Source: CAD feature listing. Evaluate the final solid. Frame: model axes, mm. Face numbers are marked on the shaded views. A direction names the side the tool comes from. Coordinates: 2 decimals unless noted, no trailing zeros. Write each loop counter-clockwise with the first axis right and the second up, starting at its lowest first coordinate (ties: lowest second). Pieces come first, ordered by that corner, then holes. Notation, with made-up numbers: M 42,26.25 L 74,26.25 A26 cw 74,50.25 Z; hole C 3,-30 d6. An arc over 180 degrees is marked long. One line per item, written item: value. Start each with the question number.
Item 1: Cut plane A-A, the plane z = 5.5. Output: boundary loops of the cut face in (x, y), then the cut area to 3 significant figures.
Item 2: Set-up query: the marked faces 1, 2, 3 and 4. Return all of +Z, -Z, +X, -X, +Y, -Y with unobstructed straight access to the full face (end or side cutting, diameter ignored); none if empty.
Item 3: Ray query, L1, parallel to X at y = 5.4, z = -7.5; L2, parallel to X at y = 4.3, z = 17.25; L3, parallel to Z at x = 0.5, y = 2.9. Return the intervals inside material, ascending. Write a range as from..to.
Item 4: Pin query (flat end, axial travel): P1, Ø3, axis at y = 5, z = -7, coming from the -X side; P2, Ø0.5, axis at x = -0.5, y = 5, coming from the -Z side; P3, Ø1.3, axis at y = 4.5, z = 1, coming from the +X side. Return the tip coordinate at first contact, or that it passes through.
Item 5: Cut plane C-C, the plane z = -4. Output: boundary loops of the cut face in (x, y).
Item 6: Cut plane B-B, the plane x = 3. Output: boundary loops of the cut face in (y, z), then the cut area to 3 significant figures.
```python
from build123d import *

# Parameters (mm, degrees)
SKETCH1_W           = 15.5
SKETCH1_H           = 11
BOSS_EXTRUDE1_DEPTH = 1.6
BOSS_EXTRUDE2_DEPTH = 1.6
SKETCH3_W           = 40.5
SKETCH3_H           = 21
BOSS_EXTRUDE3_DEPTH = 6
CUT_EXTRUDE1_DEPTH  = 2.6
SKETCH5_W           = 5
SKETCH5_H           = 4
BOSS_EXTRUDE4_DEPTH = 6
LPATTERN1_COUNT     = 2
LPATTERN1_PITCH     = 15
LPATTERN1_COL_COUNT = 2
LPATTERN1_COL_PITCH = 15
SKETCH6_W           = 4
SKETCH6_H           = 5
BOSS_EXTRUDE5_DEPTH = 6
SKETCH7_W           = 2.75
SKETCH7_H           = 4
BOSS_EXTRUDE6_DEPTH = 6


with BuildPart() as part:
    # Sketch1 → Boss-Extrude1 (new body)
    with BuildSketch(Plane(origin=(0, 0, 0), x_dir=(1, 0, 0), z_dir=(0, 1, 0))):
        with Locations((7.75, -5.5)):
            Rectangle(SKETCH1_W, SKETCH1_H)
    extrude(amount=BOSS_EXTRUDE1_DEPTH)

    # Sketch2 → Boss-Extrude2 (add, through all)
    with BuildSketch(Plane(origin=(0, 1.6, 0), x_dir=(1, 0, 0), z_dir=(0, 1, 0))):
        with BuildLine():
            Line((-1.75, -4), (-1.75, -2.6))
            ThreePointArc((-1.75, -2.6), (-4.65, -5.5), (-1.75, -8.4))
            Line((-1.75, -8.4), (-1.75, -7))
            ThreePointArc((-1.75, -7), (-3.25, -5.5), (-1.75, -4))
        make_face()
        with BuildLine():
            ThreePointArc((0, -3.187533784), (-0.827002716, -2.750804479), (-1.75, -2.6))
            Line((-1.75, -2.6), (-1.75, -4))
            ThreePointArc((-1.75, -4), (-0.689339828, -4.439339828), (-0.25, -5.5))
            ThreePointArc((-0.25, -5.5), (-0.689339828, -6.560660172), (-1.75, -7))
            Line((-1.75, -7), (-1.75, -8.4))
            ThreePointArc((-1.75, -8.4), (-0.827002716, -8.249195521), (0, -7.812466216))
            Line((0, -7.812466216), (0, -3.187533784))
        make_face()
        with BuildLine():
            Line((0, -2.6), (-1.75, -2.6))
            ThreePointArc((-1.75, -2.6), (-0.827002716, -2.750804479), (0, -3.187533784))
            Line((0, -3.187533784), (0, -2.6))
        make_face()
        with BuildLine():
            ThreePointArc((0, -7.812466216), (-0.827002716, -8.249195521), (-1.75, -8.4))
            Line((-1.75, -8.4), (0, -8.4))
            Line((0, -8.4), (0, -7.812466216))
        make_face()
        with BuildLine():
            ThreePointArc((20.15, -5.5), (19.300609665, -3.449390335), (17.25, -2.6))
            Line((17.25, -2.6), (17.25, -4))
            ThreePointArc((17.25, -4), (18.310660172, -4.439339828), (18.75, -5.5))
            ThreePointArc((18.75, -5.5), (18.310660172, -6.560660172), (17.25, -7))
            Line((17.25, -7), (17.25, -8.4))
            ThreePointArc((17.25, -8.4), (19.300609665, -7.550609665), (20.15, -5.5))
        make_face()
        with BuildLine():
            Line((17.25, -4), (17.25, -2.6))
            ThreePointArc((17.25, -2.6), (16.327002716, -2.750804479), (15.5, -3.187533784))
            Line((15.5, -3.187533784), (15.5, -7.812466216))
            ThreePointArc((15.5, -7.812466216), (16.327002716, -8.249195521), (17.25, -8.4))
            Line((17.25, -8.4), (17.25, -7))
            ThreePointArc((17.25, -7), (15.75, -5.5), (17.25, -4))
        make_face()
        with BuildLine():
            Line((17.25, -2.6), (15.5, -2.6))
            Line((15.5, -2.6), (15.5, -3.187533784))
            ThreePointArc((15.5, -3.187533784), (16.327002716, -2.750804479), (17.25, -2.6))
        make_face()
        with BuildLine():
            Line((15.5, -7.812466216), (15.5, -8.4))
            Line((15.5, -8.4), (17.25, -8.4))
            ThreePointArc((17.25, -8.4), (16.327002716, -8.249195521), (15.5, -7.812466216))
        make_face()
    extrude(amount=-BOSS_EXTRUDE2_DEPTH)

    # Sketch4 → Cut-Extrude1 (cut, through all)
    with BuildSketch(Plane(origin=(0, 1.6, 0), x_dir=(1, 0, 0), z_dir=(0, 1, 0))):
        with BuildLine():
            Line((0, 0), (0, -2.6))
            Line((0, -2.6), (-1.75, -2.6))
            ThreePointArc((-1.75, -2.6), (-4.65, -5.5), (-1.75, -8.4))
            Line((-1.75, -8.4), (0, -8.4))
            Line((0, -8.4), (0, -11))
            Line((0, -11), (15.5, -11))
            Line((15.5, -11), (15.5, -8.4))
            Line((15.5, -8.4), (17.25, -8.4))
            ThreePointArc((17.25, -8.4), (20.15, -5.5), (17.25, -2.6))
            Line((17.25, -2.6), (15.5, -2.6))
            Line((15.5, -2.6), (15.5, 0))
            Line((15.5, 0), (0, 0))
        make_face()
    extrude(amount=-CUT_EXTRUDE1_DEPTH, mode=Mode.SUBTRACT)


with BuildPart() as body_2:
    # Sketch3 → Boss-Extrude3 (new body)
    with BuildSketch(Plane(origin=(0, 1.6, 0), x_dir=(1, 0, 0), z_dir=(0, 1, 0))):
        with Locations((7.75, -5.5)):
            Rectangle(SKETCH3_W, SKETCH3_H)
        with BuildLine():
            Line((0, 0), (0, -2.6))
            Line((0, -2.6), (-1.75, -2.6))
            ThreePointArc((-1.75, -2.6), (-4.65, -5.5), (-1.75, -8.4))
            Line((-1.75, -8.4), (0, -8.4))
            Line((0, -8.4), (0, -11))
            Line((0, -11), (15.5, -11))
            Line((15.5, -11), (15.5, -8.4))
            Line((15.5, -8.4), (17.25, -8.4))
            ThreePointArc((17.25, -8.4), (20.15, -5.5), (17.25, -2.6))
            Line((17.25, -2.6), (15.5, -2.6))
            Line((15.5, -2.6), (15.5, 0))
            Line((15.5, 0), (0, 0))
        make_face(mode=Mode.SUBTRACT)
    extrude(amount=BOSS_EXTRUDE3_DEPTH)

    # Sketch5 → Boss-Extrude4 (add, through all)
    with BuildSketch(Plane(origin=(0, 7.6, 0), x_dir=(1, 0, 0), z_dir=(0, 1, 0))):
        with Locations((7.75, 7)):
            Rectangle(SKETCH5_W, SKETCH5_H)
        with Locations((7.75, -18)):
            Rectangle(SKETCH5_W, SKETCH5_H)
    boss_extrude4 = extrude(amount=-BOSS_EXTRUDE4_DEPTH)

    # LPattern1: Boss-Extrude4 ×2
    with Locations(*[(i * LPATTERN1_PITCH, 0, 0) for i in range(1, LPATTERN1_COUNT)]):
        add(boss_extrude4)

    # LPattern1 col: Boss-Extrude4 ×2
    with Locations(*[(-i * LPATTERN1_COL_PITCH, 0, 0) for i in range(1, LPATTERN1_COL_COUNT)]):
        add(boss_extrude4)

    # Sketch6 → Boss-Extrude5 (add, through all)
    with BuildSketch(Plane(origin=(0, 7.6, 0), x_dir=(1, 0, 0), z_dir=(0, 1, 0))):
        with Locations((-14.5, -5.5)):
            Rectangle(SKETCH6_W, SKETCH6_H)
        with Locations((30, -5.5)):
            Rectangle(SKETCH6_W, SKETCH6_H)
    extrude(amount=-BOSS_EXTRUDE5_DEPTH)

    # Sketch7 → Boss-Extrude6 (add, through all)
    with BuildSketch(Plane(origin=(0, 1.6, 0), x_dir=(-1, 0, 0), z_dir=(0, -1, 0))):
        with Locations((11.125, -18)):
            Rectangle(SKETCH7_W, SKETCH7_H)
        with Locations((-26.625, -18)):
            Rectangle(SKETCH7_W, SKETCH7_H)
    extrude(amount=-BOSS_EXTRUDE6_DEPTH)


solid = body_2.part
```
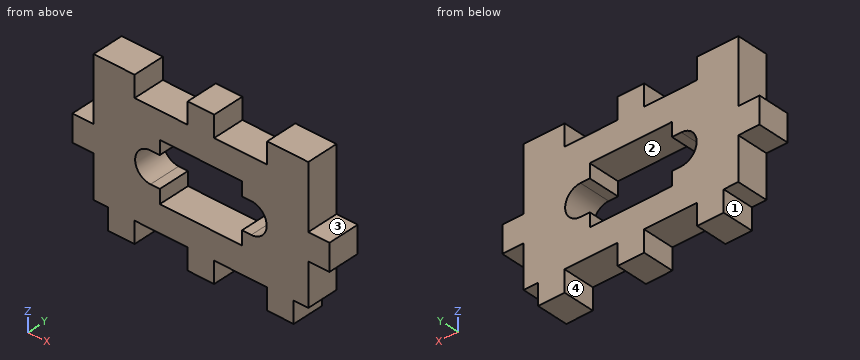
From the geometry:
1. outline: M -16.5,1.6 L -4.65,1.6 L -4.65,7.6 L -16.5,7.6 Z; M 20.15,1.6 L 32,1.6 L 32,7.6 L 20.15,7.6 Z
1. area: 142 mm²
2. face 1: -Z, -X, +Y, -Y
2. face 2: +Y, -Y
2. face 3: +Z, +X, +Y, -Y
2. face 4: -Z, +Y, -Y
3. L1: x = -9.75..-4.75, 5.25..10.25, 20.25..25.25
3. L2: x = -12.5..-4.75, 5.25..10.25, 20.25..28
3. L3: z = -5..0, 11..16
4. P1: stops at x = -9.75
4. P2: stops at z = -5
4. P3: stops at x = 28
5. outline: M -12.5,1.6 L 28,1.6 L 28,7.6 L -12.5,7.6 Z
6. outline: M 1.6,-5 L 7.6,-5 L 7.6,0 L 1.6,0 Z; M 1.6,11 L 7.6,11 L 7.6,16 L 1.6,16 Z
6. area: 60.0 mm²
